```python
from build123d import *

# Parameters (mm, degrees)
F1_DEPTH = 63.5
F2_DEPTH = 25.4
F3_DEPTH = 7.9375
F5_R     = 6.35


# Not quite as in the source:
# - a feature names something its author has since deleted; it is built from what else it names


with BuildPart() as f1:
    # F0 (on Front) → F1 (new body, symmetric)
    with BuildSketch(Plane.XZ):
        Polygon((22.225, 9.525), (-41.275, 9.525), (-41.275, -9.525), (41.275, -9.525), (41.275, 9.525), align=None)
    extrude(amount=F1_DEPTH, both=True)

    # F0 (on Front) → F2 (join, symmetric)
    with BuildSketch(Plane.XZ):
        with BuildLine():
            Line((85.725, 61.9848461288), (60.325, 61.9848461288))
            Line((60.325, 61.9848461288), (57.15, 61.9848461288))
            add(Edge.make_bspline(
                [(55.8188394438, 61.9594684272), (56.2631889725, 61.9701778386), (56.7069273587, 61.9786434716), (57.15, 61.9848461288)],
                knots=[110.4431341751, 110.4431341751, 110.4431341751, 110.4431341751, 111.5325785628, 111.5325785628, 111.5325785628, 111.5325785628], degree=3))
            ThreePointArc((55.8188394438, 61.9594684272), (31.9880604143, 51.2803420215), (22.225, 27.0598461288))
            Line((22.225, 27.0598461288), (22.225, 9.525))
            Line((22.225, 9.525), (41.275, 9.525))
            Line((41.275, 9.525), (41.275, 27.0598461288))
            ThreePointArc((41.275, 27.0598461288), (45.9246798487, 38.2851662801), (57.15, 42.9348461288))
            Line((57.15, 42.9348461288), (60.325, 42.9348461288))
            Line((60.325, 42.9348461288), (85.725, 42.9348461288))
            Line((85.725, 42.9348461288), (85.725, 61.9848461288))
        make_face()
    extrude(amount=F2_DEPTH, both=True)

    # F0 (on Front) → F3 (join, symmetric)
    with BuildSketch(Plane.XZ):
        with BuildLine():
            ThreePointArc((22.225, 27.0598461288), (31.9880604143, 51.2803420215), (55.8188394438, 61.9594684272))
            add(Edge.make_bspline(
                [(-41.275, 9.525), (-40.5543307974, 36.728759834), (10.7726166473, 60.8737948733), (55.8188394438, 61.9594684272)],
                knots=[0, 0, 0, 0, 110.4431341751, 110.4431341751, 110.4431341751, 110.4431341751], degree=3))
            Line((-41.275, 9.525), (22.225, 9.525))
            Line((22.225, 9.525), (22.225, 27.0598461288))
        make_face()
    extrude(amount=F3_DEPTH, both=True)

    # F0 (on Front) → F4 (revolve)
    with BuildSketch(Plane.XZ):
        Polygon((111.125, 66.675), (85.725, 66.675), (85.725, 61.9848461288), (85.725, 42.9348461288), (85.725, 38.1), (111.125, 38.1), align=None)
    revolve(axis=Axis((85.725, 0, 52.3875), (0, 0, 1)))

    # F5
    f5_edges = [f1.edges().sort_by_distance(p)[0] for p in [
        (41.275, -63.5, 0),
        (-41.275, -63.5, 0),
        (-41.275, 63.5, 0),
        (41.275, 63.5, 0),
    ]]
    fillet(f5_edges, radius=F5_R)


solid = f1.part
```
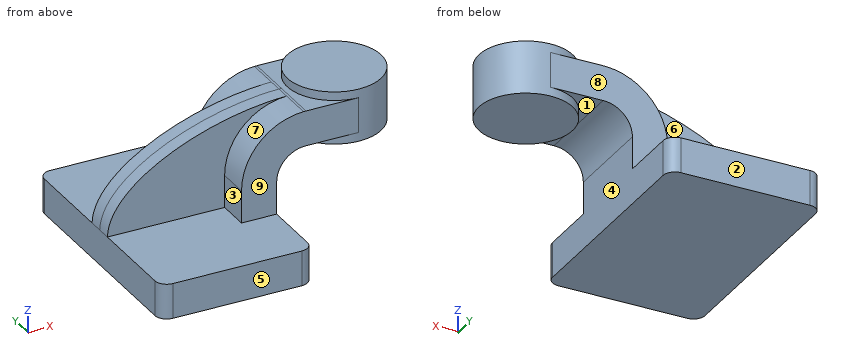
Design review of the part built by this model. Coordinates are the model's own, in mm. Face numbers are marked on the shaded views. A direction names the side the tool comes from. Give positions to 0.01 mm unless a question says otherwise; leave off trailing zeros. Loops run counter-clockwise (first coordinate to the right, second up) from the corner with the lowest first, then second, coordinate; pieces in that order, holes last. Notation, with made-up numbers: (63, -27) -> (68, -27) arc R25 ccw to (68, -14) -> close; hole circle Ø4 at (76, -3.75). An arc over 180 degrees is marked (long way). Write each question's results on one line, items separated by ' | '.
Q1. Take a section at D-D, the plane x = 100.5. Write out the cut boundary in (y, z) (3 decimals), plus the area to 3 significant figures.
Reply:
outline: (-20.661, 38.1) -> (20.661, 38.1) -> (20.661, 66.675) -> (-20.661, 66.675) -> close | area: 1,180 mm²
Q2. For pin 1 Ø8.5 at (y, z) = (-20.5, 21) entering from -X (3 decimals); pin 2 Ø16.5 at (x, y) = (-12, -46.5) entering from +Z (3 decimals); pin 3 Ø1.5 at (y, z) = (-16.5, -1.5) entering from +X (3 decimals), all flat-tipped, find the tip position at first contact; note any pin that passes through.
Reply:
pin 1: stops at x = 22.225 | pin 2: stops at z = 9.525 | pin 3: stops at x = 41.275
Q3. Take a section at B-B, the plane x = 72. Write out the cut boundary in (y, z) (3 decimals), plus the area to 3 significant figures.
Reply:
outline: (-25.4, 42.935) -> (-21.373, 42.935) -> (-21.373, 38.1) -> (21.373, 38.1) -> (21.373, 42.935) -> (25.4, 42.935) -> (25.4, 61.985) -> (21.373, 61.985) -> (21.373, 66.675) -> (-21.373, 66.675) -> (-21.373, 61.985) -> (-25.4, 61.985) -> close | area: 1,370 mm²
Q4. Take a section at C-C, the plane y = 32.5. Write out the cut boundary in (x, z) (3 decimals).
Reply:
outline: (-41.275, -9.525) -> (41.275, -9.525) -> (41.275, 9.525) -> (-41.275, 9.525) -> close
Q5. Wall thickness on L1, parallel to Y at x = 10.5, z = 45; L2, parallel to Y at x = 55.5, z = 54.5; L3, parallel to X at y = 52, z = 9 (3 decimals): over which ranges is each line inside the solid? List them lowest first.
Reply:
L1: y = -7.94 to 7.94 | L2: y = -25.4 to 25.4 | L3: x = -41.275 to 41.275
Q6. The part is to be moulded in two halves that separate along X. For the marked faces 1, 2, 3 and 4, say which applies: +X half, -X half, draft (parallel to the pull), parting line (faces both ways), or undercut.
Reply:
face 1: undercut | face 2: draft | face 3: -X half | face 4: +X half
Q7. Machinability: for the marked faces 5, 6, 7, 8 and 9, which of the approach directions +Z, -Z, +X, -X, +Y, -Y give a long, thin tool a straight path to every point of the face, cutting with its end or side? Answer none if there is none.
Reply:
face 5: +Z, -Z, +X, -X, -Y | face 6: +Z, -X, +Y | face 7: +Z, -X, -Y | face 8: +Z, +X, -X, +Y | face 9: +Z, +X, -X, -Y
Q8. Take a section at A-A, the plane z = -3.5. Write out the cut boundary in (x, y) (3 decimals), plus the area to 3 significant figures.
Reply:
outline: (-41.275, -57.15) arc R6.35 ccw to (-34.925, -63.5) -> (34.925, -63.5) arc R6.35 ccw to (41.275, -57.15) -> (41.275, 57.15) arc R6.35 ccw to (34.925, 63.5) -> (-34.925, 63.5) arc R6.35 ccw to (-41.275, 57.15) -> close | area: 10,400 mm²
